Could you check a few things on this model? Use its own coordinates, in mm. Face numbers are marked on the shaded views. A direction names the side the tool comes from. Coordinates: 2 decimals unless noted, no trailing zeros. Order: outer loops, then holes, each group sorted by start corner. A loop starts at its lowest first (then second) coordinate and runs counter-clockwise, first axis right, second up. Notation, with made-up numbers: (-6.5, 48.5) - (44.5, 48.5) arc R18 ccw to (44.5, 56.5) - close; hole circle Ø2 at (36, 67). An arc over 180 degrees is marked (long way). One line per item, written item: value. Start each with the question number.
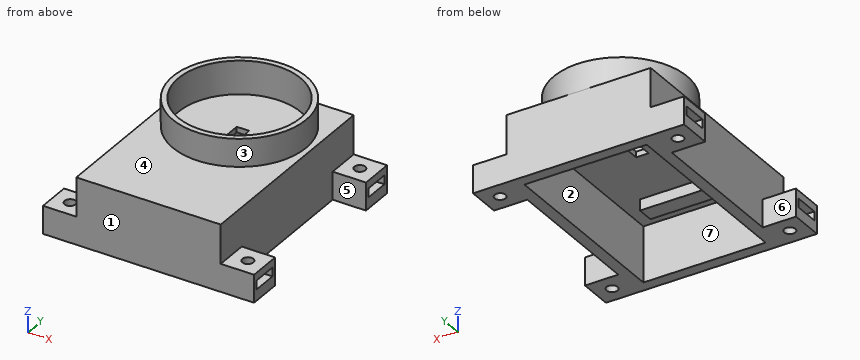
from build123d import *

# Parameters (mm, degrees)
SKETCH_1_W          = 26
SKETCH_1_H          = 38
EXTRUDE_1_DEPTH     = 12
SKETCH_2_W          = 22
SKETCH_2_H          = 34
CUT_EXTRUDE_1_DEPTH = 10
SKETCH_3_W          = 2.25
SKETCH_3_H          = 7.25
CUT_EXTRUDE_3_DEPTH = 12
SKETCH_4_W          = 6
SKETCH_4_H          = 6
EXTRUDE_2_DEPTH     = 5
SKETCH_5_R          = 1
CUT_EXTRUDE_4_DEPTH = 13
CUT_EXTRUDE_START   = 2
CUT_EXTRUDE_5_DEPTH = 1.6
SKETCH_7_R          = 12
SKETCH_7_R_2        = 11
EXTRUDE_3_DEPTH     = 5
SKETCH_9_R          = 11
CUT_EXTRUDE_7_DEPTH = 1
SKETCH_10_W         = 14.41096837
SKETCH_10_H         = 3
EXTRUDE_4_DEPTH     = 2
CUT_EXTRUDE_START_2 = 20
SKETCH_11_W         = 1.6
SKETCH_11_H         = 4.5
CUT_EXTRUDE_8_DEPTH = 4
CUT_EXTRUDE_START_3 = -20
SKETCH_13_W         = 1.6
SKETCH_13_H         = 4.5
CUT_EXTRUDE_9_DEPTH = 4


with BuildPart() as part:
    # ｽｹｯﾁ1 → ﾎﾞｽ - 押し出し1 (new body)
    with BuildSketch(Plane.XY):
        Rectangle(SKETCH_1_W, SKETCH_1_H)
    extrude(amount=EXTRUDE_1_DEPTH)

    # ｽｹｯﾁ2 → ｶｯﾄ - 押し出し1 (cut)
    with BuildSketch(Plane.XY):
        Rectangle(SKETCH_2_W, SKETCH_2_H)
    extrude(amount=CUT_EXTRUDE_1_DEPTH, mode=Mode.SUBTRACT)

    # ｽｹｯﾁ3 → ｶｯﾄ - 押し出し3 (cut)
    with BuildSketch(Plane.XY):
        with Locations((0, 4.375)):
            Rectangle(SKETCH_3_W, SKETCH_3_H)
    extrude(amount=CUT_EXTRUDE_3_DEPTH, mode=Mode.SUBTRACT)

    # ｽｹｯﾁ4 → ﾎﾞｽ - 押し出し2 (add)
    with BuildSketch(Plane.XY):
        with Locations((16, 16)):
            Rectangle(SKETCH_4_W, SKETCH_4_H)
        with Locations((16, -16)):
            Rectangle(SKETCH_4_W, SKETCH_4_H)
        with Locations((-16, -16)):
            Rectangle(SKETCH_4_W, SKETCH_4_H)
        with Locations((-16, 16)):
            Rectangle(SKETCH_4_W, SKETCH_4_H)
    extrude(amount=EXTRUDE_2_DEPTH)

    # ｽｹｯﾁ5 → ｶｯﾄ - 押し出し4 (cut, through all)
    with BuildSketch(Plane.XY):
        with Locations((-16, 16)):
            Circle(SKETCH_5_R)
        with Locations((-16, -16)):
            Circle(SKETCH_5_R)
        with Locations((16, -16)):
            Circle(SKETCH_5_R)
        with Locations((16, 16)):
            Circle(SKETCH_5_R)
    extrude(amount=CUT_EXTRUDE_4_DEPTH, mode=Mode.SUBTRACT)

    # ｽｹｯﾁ6 → ｶｯﾄ - 押し出し5 (cut)
    with BuildSketch(Plane.XY.offset(CUT_EXTRUDE_START)):
        Polygon((-17.184124892, 17.98272075), (-18.309148984, 15.965878137), (-17.125024092, 13.983157387), (-14.815875108, 14.01727925), (-13.690851016, 16.034121863), (-14.874975908, 18.016842613), align=None)
        Polygon((-17.07560545, -13.956374239), (-18.307634549, -15.909688764), (-17.2320291, -17.953314524), (-14.92439455, -18.043625761), (-13.692365451, -16.090311236), (-14.7679709, -14.046685476), align=None)
        Polygon((14.939341307, 18.051423035), (13.693086191, 16.107154145), (14.753744884, 14.055731109), (17.060658693, 13.948576965), (18.306913809, 15.892845855), (17.246255116, 17.944268891), align=None)
        Polygon((14.854466591, -13.994735294), (13.690623119, -15.98942868), (14.836156527, -17.994693386), (17.145533409, -18.005264706), (18.309376881, -16.01057132), (17.163843473, -14.005306614), align=None)
    extrude(amount=CUT_EXTRUDE_5_DEPTH, mode=Mode.SUBTRACT)

    # ｽｹｯﾁ7 → ﾎﾞｽ - 押し出し3 (add)
    with BuildSketch(Plane.XY.offset(12)):
        with Locations((0, 7)):
            Circle(SKETCH_7_R)
        with Locations((0, 7)):
            Circle(SKETCH_7_R_2, mode=Mode.SUBTRACT)
    extrude(amount=EXTRUDE_3_DEPTH)

    # ｽｹｯﾁ9 → ｶｯﾄ - 押し出し7 (cut)
    with BuildSketch(Plane.XY.offset(12)):
        with Locations((0, 7)):
            Circle(SKETCH_9_R)
    extrude(amount=-CUT_EXTRUDE_7_DEPTH, mode=Mode.SUBTRACT)

    # ｽｹｯﾁ10 → ﾎﾞｽ - 押し出し4 (add)
    with BuildSketch(Plane.XY.offset(10)):
        with Locations((0, -11.5)):
            Rectangle(SKETCH_10_W, SKETCH_10_H)
    extrude(amount=-EXTRUDE_4_DEPTH)

    # ｽｹｯﾁ11 → ｶｯﾄ - 押し出し8 (cut)
    with BuildSketch(Plane(origin=(0, 0, 0), x_dir=(0, 0, -1), z_dir=(1, 0, 0)).offset(CUT_EXTRUDE_START_2)):
        with Locations((-2.8, 16)):
            Rectangle(SKETCH_11_W, SKETCH_11_H)
        with Locations((-2.8, -16)):
            Rectangle(SKETCH_11_W, SKETCH_11_H)
    extrude(amount=-CUT_EXTRUDE_8_DEPTH, mode=Mode.SUBTRACT)

    # ｽｹｯﾁ13 → ｶｯﾄ - 押し出し9 (cut)
    with BuildSketch(Plane(origin=(0, 0, 0), x_dir=(0, 0, -1), z_dir=(1, 0, 0)).offset(CUT_EXTRUDE_START_3)):
        with Locations((-2.8, 16)):
            Rectangle(SKETCH_13_W, SKETCH_13_H)
        with Locations((-2.8, -16)):
            Rectangle(SKETCH_13_W, SKETCH_13_H)
    extrude(amount=CUT_EXTRUDE_9_DEPTH, mode=Mode.SUBTRACT)


solid = part.part
Q1. I want a section at B-B on y = 7. Please give me the cut outline in (x, z) (3 decimals).
Q2. I want a section at A-A on z = 9.5. Please give me the cut outline in (x, y).
Q3. I want a section at D-D on z = 1.25. Please give me the cut outline in (x, y), then the cut area to 3 significant figures.
Q4. I'm going to push flat-ended pins straight in: pin 1 (1 mm diameter, centred on y = 9.5, z = 6.5, fed in from +X); pin 2 (3 mm diameter, centred on x = 15.5, y = -15.5, fed in from +Z); pin 3 (0.9 mm diameter, centred on x = 2.5, y = -11.5, fed in from -Z). Where does each tip first touch, or does it pass through?
Q5. Which directions (+Z, -Z, +X, -X, +Y, -Y) give clear straight access to the entire face, cutting with the end or side of a thin tool? Please do the marked faces 4, 5, 6 and 7.
Q6. If I drill on L1, parallel to Y at x = -16, z = 1.4; L2, parallel to X at y = -16, z = 4; L3, parallel to Y at x = 5, z = 9.75, over which ranges is the centre line in solid material (lowest first)?
Q7. I want a section at C-C on z = 7. Please give me the cut outline in (x, y), then the cut area to 3 significant figures.
Q8. We'd pull the mould along X, two halves only. Please class the marked faces 1, 2 and 3: +X half, -X half, draft (parallel to the pull), parting line (faces both ways), or undercut.
Values follow:
1. outline: (-13, 0) - (-11, 0) - (-11, 10) - (-1.125, 10) - (-1.125, 11) - (-11, 11) - (-11, 17) - (-12, 17) - (-12, 12) - (-13, 12) - close; (1.125, 10) - (11, 10) - (11, 0) - (13, 0) - (13, 12) - (12, 12) - (12, 17) - (11, 17) - (11, 11) - (1.125, 11) - close
2. outline: (-13, -19) - (13, -19) - (13, 19) - (-13, 19) - close; (-7.21, -13) - (7.21, -13) - (7.21, -10) - (-7.21, -10) - close; hole (-11, -17) - (11, -17) - (11, 17) - (-11, 17) - close
3. outline: (-19, -19) - (19, -19) - (19, -13) - (13, -13) - (13, 13) - (19, 13) - (19, 19) - (-19, 19) - (-19, 13) - (-13, 13) - (-13, -13) - (-19, -13) - close; hole circle Ø2 at (-16, -16); hole circle Ø2 at (-16, 16); hole (-11, -17) - (11, -17) - (11, 17) - (-11, 17) - close; hole circle Ø2 at (16, -16); hole circle Ø2 at (16, 16)
3. area: 371 mm^2
4. pin 1: stops at x = 13
4. pin 2: stops at z = 5
4. pin 3: stops at z = 8
5. face 4: +Z
5. face 5: +Z, -Z, +X
5. face 6: +Z, -Z, -X
5. face 7: -Z
6. L1: y = -19 to -17, -15 to -13, 13 to 15, 17 to 19
6. L2: x = -19 to -17, -15 to -11, 11 to 15, 17 to 19
6. L3: y = -19 to -17, -13 to -10, 17 to 19
7. outline: (-13, -19) - (13, -19) - (13, 19) - (-13, 19) - close; hole (-11, -17) - (11, -17) - (11, 17) - (-11, 17) - close
7. area: 240 mm^2
8. face 1: draft
8. face 2: undercut
8. face 3: parting line
